Design review of the part shown in the three views and the two pictorial views. Dimensions are in mm from the part's minimum x, y and z. A direction names the side the tool comes from. Round coordinates to 2 decimals unless told otherwise and drop trailing zeros. Loops run counter-clockwise (first coordinate to the right, second up) from the corner with the lowest first, then second, coordinate; pieces in that order, holes last.
1. Tool access review of the marked faces 4 and 5: name each direction out of +Z, -Z, +X, -X, +Y, -Y from which nothing blocks a thin tool from reaching the whole face with its end or side.
2. Clearance check with flat-ended pins moving along their axes: pin 1 Ø1 at (x, y) = (4, 8.5) entering from +Z; pin 2 Ø2 at (x, y) = (9, 8) entering from +Z; pin 3 Ø1.5 at (y, z) = (8, 10) entering from -X. State where each tip first meets the part, or that it passes through.
3. Consider section D-D on y = 1.5. State the section outline as (x, z) points (3 decimals), then the cut area to 3 significant figures.
4. To check wall thickness, follow line 1 along Z through (x, y) = (9, 13.75) (3 decimals); line 2 along X through (y, z) = (4.25, 9.25). State the ranges of each line that lie inside material, in increasing order.
5. Consider section C-C on y = 17. State the section outline as (x, z) points (3 decimals), then the cut area to 3 significant figures.
6. Draft analysis for pull direction Z (two halves, no side actions). For the marked faces 1, 2 and 3, state which applies: released by +Z, released by -Z, zero draft, split by the parting line, or undercut.
7. Consider section A-A on x = 9. State the section outline as (y, z) points (3 decimals), then the cut area to 3 significant figures.
8. Consider section B-B on z = 9. State the section outline as (x, y) points (3 decimals), then the cut area to 3 significant figures.
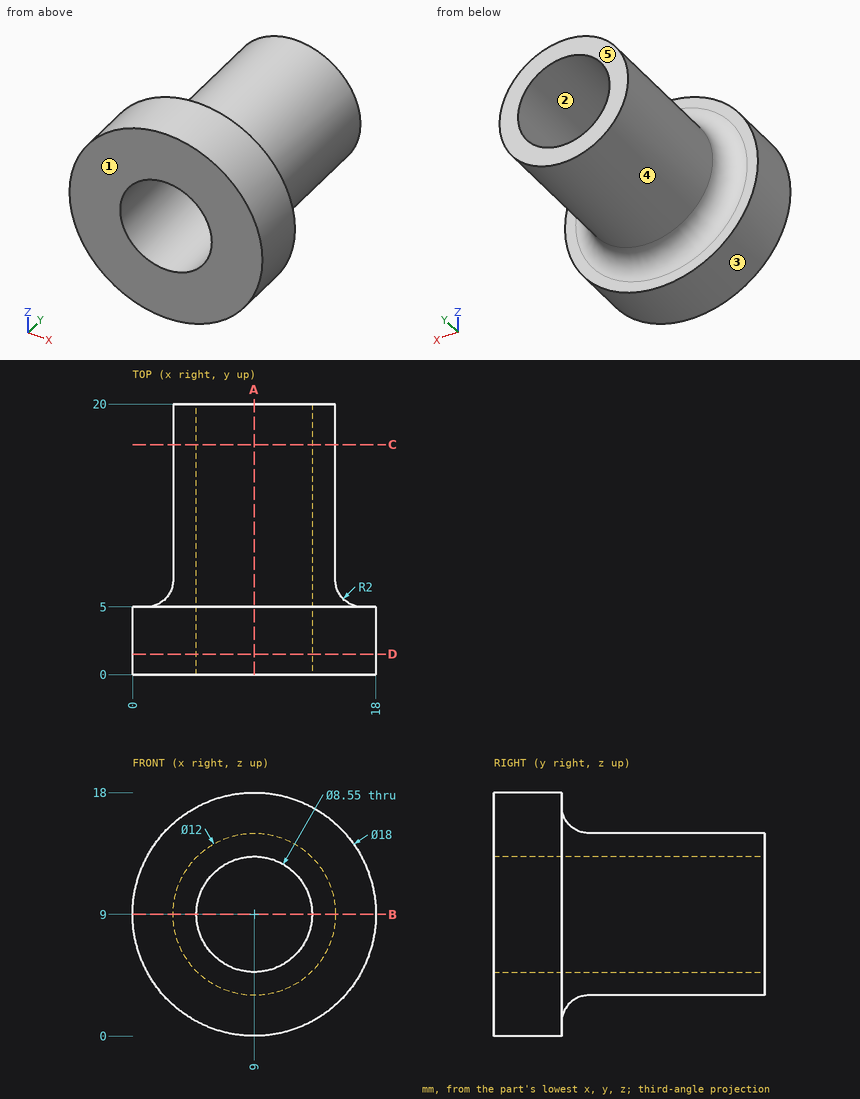
Resolved:
1. face 4: +Y
1. face 5: +Z, -Z, +X, -X, +Y
2. pin 1: stops at z = 12.97
2. pin 2: stops at z = 15
2. pin 3: stops at x = 3.01
3. outline: circle Ø18 at (9, 9); hole circle Ø8.55 at (9, 9)
3. area: 197 mm2
4. line 1: z = 3 to 4.725, 13.275 to 15
4. line 2: x = 0 to 4.73, 13.27 to 18
5. outline: circle Ø12 at (9, 9); hole circle Ø8.55 at (9, 9)
5. area: 55.7 mm2
6. face 1: zero draft
6. face 2: undercut
6. face 3: split by the parting line
7. outline: (0, 0) - (5, 0) - (5, 1) arc R2 cw to (7, 3) - (20, 3) - (20, 4.725) - (0, 4.725) - close; (0, 13.275) - (20, 13.275) - (20, 15) - (7, 15) arc R2 cw to (5, 17) - (5, 18) - (0, 18) - close
7. area: 101 mm2
8. outline: (0, 0) - (4.725, 0) - (4.725, 20) - (3, 20) - (3, 7) arc R2 cw to (1, 5) - (0, 5) - close; (13.275, 0) - (18, 0) - (18, 5) - (17, 5) arc R2 cw to (15, 7) - (15, 20) - (13.275, 20) - close
8. area: 101 mm2
